```python
from build123d import *

# Parameters (mm, degrees)
ESQUISSE1_W               = 43.3
ESQUISSE1_H               = 43.3
BOSS_EXTRU_1_DEPTH        = 1.6
ESQUISSE2_R               = 1.75
ENL_V_MAT_EXTRU_1_DEPTH   = 62.25634661
SYM_TRIE2_COPY_1_SKETCH_R = 1.75
SYM_TRIE2_COPY_1_DEPTH    = 62.25634661


with BuildPart() as part:
    # Esquisse1 → Boss.-Extru.1 (new body)
    with BuildSketch(Plane.XY):
        with Locations((21.65, 21.65)):
            Rectangle(ESQUISSE1_W, ESQUISSE1_H)
    extrude(amount=BOSS_EXTRU_1_DEPTH)

    # Esquisse2 → Enlèv. mat.-Extru.1 (cut, through all)
    with BuildSketch(Plane.XY.offset(1.6)):
        with Locations((3.45, 39.85)):
            Circle(ESQUISSE2_R)
    enl_v_mat_extru_1 = extrude(amount=-ENL_V_MAT_EXTRU_1_DEPTH, mode=Mode.SUBTRACT)

    # Symétrie1: Enlèv. mat.-Extru.1 across plane
    add(enl_v_mat_extru_1.mirror(Plane.ZY.offset(-21.65)), mode=Mode.SUBTRACT)

    # Symétrie2: Enlèv. mat.-Extru.1 across plane
    add(enl_v_mat_extru_1.mirror(Plane.ZX.offset(21.65)), mode=Mode.SUBTRACT)

    # Symétrie2 copy 1 sketch → Symétrie2 copy 1 (cut, through all)
    with BuildSketch(Plane(origin=(43.3, 43.3, 1.6), x_dir=(-1, 0, 0), z_dir=(0, 0, 1))):
        with Locations((3.45, 39.85)):
            Circle(SYM_TRIE2_COPY_1_SKETCH_R)
    extrude(amount=-SYM_TRIE2_COPY_1_DEPTH, mode=Mode.SUBTRACT)


solid = part.part
```
The model under review builds one solid part; all positions refer to its coordinate system, in mm. Give positions to 0.01 mm unless a question says otherwise; leave off trailing zeros. Loops run counter-clockwise (first coordinate to the right, second up) from the corner with the lowest first, then second, coordinate; pieces in that order, holes last. Notation, with made-up numbers: (76.25, 31) -> (94.25, 31) arc R18 ccw to (94.25, 49) -> close; hole circle Ø7 at (76, 63). An arc over 180 degrees is marked (long way). Use CSV: the item, a comma, the result in double quotes.
1. To check wall thickness, follow probe 1 along Y at (x, z) = (39.85, 1). State the ranges of the line that lie inside material, in increasing order. Write a range as from..to.
Result:
probe 1,"y = 0..1.7, 5.2..38.1, 41.6..43.3"
2. Consider section C-C, the plane z = 0.5. Write out the cut boundary in (x, y).
Result:
outline,"(0, 0) -> (43.3, 0) -> (43.3, 43.3) -> (0, 43.3) -> close; hole circle Ø3.5 at (3.45, 3.45); hole circle Ø3.5 at (3.45, 39.85); hole circle Ø3.5 at (39.85, 3.45); hole circle Ø3.5 at (39.85, 39.85)"
3. For P1, Ø2, axis at x = 39.85, y = 3.45, coming from the -Z side, flat-tipped, find the tip position at first contact; note if it passes through.
Result:
P1,"passes through"
4. The part is to be moulded in two halves that separate along Y. For faces 1 (the face through (3.07, 38.14, 0.81)), 2 (the face through (38.233, 4.12, 0.811)), 3 (the face through (21, 43.3, 1)), 4 (the face through (43.3, 21, 1)), say which applies: +Y half, -Y half, draft (parallel to the pull), parting line (faces both ways), or undercut.
Result:
face 1,"undercut"
face 2,"undercut"
face 3,"+Y half"
face 4,"draft"
5. Consider section A-A, the plane y = 39.85. Write out the cut boundary in (x, z), then the cut area to 3 significant figures.
Result:
outline,"(0, 0) -> (1.7, 0) -> (1.7, 1.6) -> (0, 1.6) -> close; (5.2, 0) -> (38.1, 0) -> (38.1, 1.6) -> (5.2, 1.6) -> close; (41.6, 0) -> (43.3, 0) -> (43.3, 1.6) -> (41.6, 1.6) -> close"
area,"58.1 mm²"
